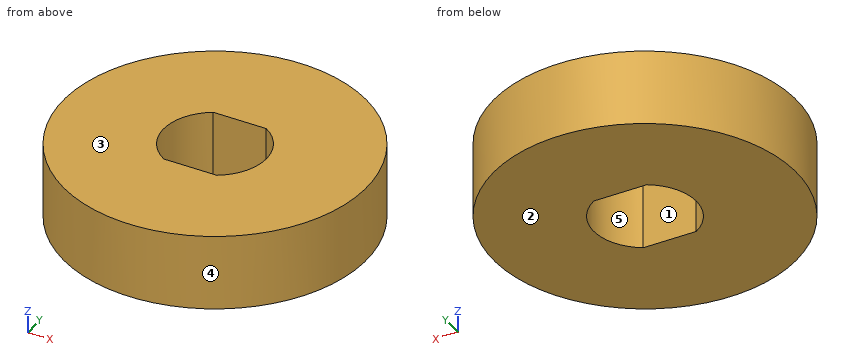
from build123d import *

# Parameters (mm, degrees)
SKETCH1_R           = 10
BOSS_EXTRUDE1_DEPTH = 5


with BuildPart() as part:
    # Sketch1 → Boss-Extrude1 (new body)
    with BuildSketch(Plane.XY):
        Circle(SKETCH1_R)
        with BuildLine():
            Line((-1.774823935, 2.9), (1.774823935, 2.9))
            ThreePointArc((1.774823935, 2.9), (3.4, 0), (1.774823935, -2.9))
            Line((1.774823935, -2.9), (-1.774823935, -2.9))
            ThreePointArc((-1.774823935, -2.9), (-3.4, 0), (-1.774823935, 2.9))
        make_face(mode=Mode.SUBTRACT)
    extrude(amount=BOSS_EXTRUDE1_DEPTH)


solid = part.part
The model under review builds one solid part; all positions refer to its coordinate system, in mm. Face numbers are marked on the shaded views. A direction names the side the tool comes from. Give positions to 0.01 mm unless a question says otherwise; leave off trailing zeros. Order: outer loops, then holes, each group sorted by start corner. A loop starts at its lowest first (then second) coordinate and runs counter-clockwise, first axis right, second up. Notation, with made-up numbers: M 54.25,68.25 L 88.25,68.25 A15 ccw 88.25,75.25 Z; hole C 5.25,34.5 d4. An arc over 180 degrees is marked long. Answer in a Markdown table with one row per item. Add a question column.
1. Add section A-A on x = 0. State the section outline as (y, z) points, plus the area to 3 significant figures.
2. Machinability: for the marked faces 1 and 2, which of the approach directions +Z, -Z, +X, -X, +Y, -Y give a long, thin tool a straight path to every point of the face, cutting with its end or side? Answer none if there is none.
3. Add section D-D on x = 5.25. State the section outline as (y, z) points.
4. Add section B-B on y = 0. State the section outline as (x, z) points, plus the area to 3 significant figures.
5. Add section C-C on z = 0.85. State the section outline as (x, y) points, plus the area to 3 significant figures.
6. For pin 1 Ø1.1 at (x, z) = (0.5, 1.5) entering from -Y; pin 2 Ø2 at (x, z) = (3, 3) entering from +Y; pin 3 Ø2 at (y, z) = (-6, 3) entering from -X; pin 4 Ø3 at (x, z) = (-7, 3.5) entering from -Y, all flat-tipped, find the tip position at first contact; note any pin that passes through.
7. Mouldability with a two-part tool opening along Y and no side actions: class the marked faces 3, 4 and 5 as released by +Y, released by -Y, zero draft, split by the parting line, or undercut.
8. To check wall thickness, follow line 1 along Y through (x, z) = (-0.25, 3.2); line 2 along X through (y, z) = (2.5, 2.65). State the ranges of each line that lie inside material, in increasing order.
The answers:
| question | item | result |
|---|---|---|
| 1 | outline | M -10,0 L -2.9,0 L -2.9,5 L -10,5 Z; M 2.9,0 L 10,0 L 10,5 L 2.9,5 Z |
| 1 | area | 71.0 mm2 |
| 2 | face 1 | +Z, -Z |
| 2 | face 2 | -Z, +X, -X, +Y, -Y |
| 3 | outline | M -8.51,0 L 8.51,0 L 8.51,5 L -8.51,5 Z |
| 4 | outline | M -10,0 L -3.4,0 L -3.4,5 L -10,5 Z; M 3.4,0 L 10,0 L 10,5 L 3.4,5 Z |
| 4 | area | 66.0 mm2 |
| 5 | outline | C 0,0 d20; hole M -1.77,-2.9 L 1.77,-2.9 A3.4 ccw 1.77,2.9 L -1.77,2.9 A3.4 ccw Z |
| 5 | area | 280 mm2 |
| 6 | pin 1 | y = -10 |
| 6 | pin 2 | y = 9.8 |
| 6 | pin 3 | x = -8.66 |
| 6 | pin 4 | y = -8.35 |
| 7 | face 3 | zero draft |
| 7 | face 4 | split by the parting line |
| 7 | face 5 | undercut |
| 8 | line 1 | -10 to -2.9, 2.9 to 10 |
| 8 | line 2 | -9.68 to -2.3, 2.3 to 9.68 |
